from build123d import *

# Parameters (mm, degrees)
EXTRUDE_1_DEPTH     = 500
CUT_EXTRUDE_1_REACH = 4
SKETCH_2_R          = 3


with BuildPart() as part:
    # 草图1 → 凸台-拉伸1 (new body)
    with BuildSketch(Plane.XY):
        with BuildLine():
            Line((0, 0), (19.917157288, 0))
            ThreePointArc((19.917157288, 0), (19.993693974, 0.015224093), (20.058578644, 0.058578644))
            Line((20.058578644, 0.058578644), (43.444365081, 23.444365081))
            ThreePointArc((43.444365081, 23.444365081), (45, 24.088730163), (46.555634919, 23.444365081))
            Line((46.555634919, 23.444365081), (69.941421356, 0.058578644))
            ThreePointArc((69.941421356, 0.058578644), (70.006306026, 0.015224093), (70.082842712, 0))
            Line((70.082842712, 0), (90, 0))
            Line((90, 0), (90, -2))
            Line((90, -2), (70.082842712, -2))
            ThreePointArc((70.082842712, -2), (69.240939161, -1.832534972), (68.527207794, -1.355634919))
            Line((68.527207794, -1.355634919), (45.141421356, 22.030151519))
            ThreePointArc((45.141421356, 22.030151519), (45, 22.088730163), (44.858578644, 22.030151519))
            Line((44.858578644, 22.030151519), (21.472792206, -1.355634919))
            ThreePointArc((21.472792206, -1.355634919), (20.759060839, -1.832534972), (19.917157288, -2))
            Line((19.917157288, -2), (0, -2))
            Line((0, -2), (0, 0))
        make_face()
    extrude(amount=EXTRUDE_1_DEPTH)

    # 草图2 → 切除-拉伸1 (cut, up to next)
    with BuildSketch(Plane(origin=(0, 0, 0), x_dir=(1, 0, 0), z_dir=(0, 1, 0)), mode=Mode.PRIVATE) as cut_extrude_1_sk1:
        with Locations((9.958578644, -20)):
            Circle(SKETCH_2_R)
    cut_extrude_1_tool1 = extrude(cut_extrude_1_sk1.sketch, amount=-CUT_EXTRUDE_1_REACH, mode=Mode.PRIVATE) & part.part
    add(cut_extrude_1_tool1.solids().sort_by_distance((9.958579, 0, 20))[0], mode=Mode.SUBTRACT)
    # 草图2 → 切除-拉伸1 (cut, up to next)
    with BuildSketch(Plane(origin=(0, 0, 0), x_dir=(1, 0, 0), z_dir=(0, 1, 0)), mode=Mode.PRIVATE) as cut_extrude_1_sk2:
        with Locations((80.041421356, -20)):
            Circle(SKETCH_2_R)
    cut_extrude_1_tool2 = extrude(cut_extrude_1_sk2.sketch, amount=-CUT_EXTRUDE_1_REACH, mode=Mode.PRIVATE) & part.part
    add(cut_extrude_1_tool2.solids().sort_by_distance((80.041421, 0, 20))[0], mode=Mode.SUBTRACT)
    # 草图2 → 切除-拉伸1 (cut, up to next)
    with BuildSketch(Plane(origin=(0, 0, 0), x_dir=(1, 0, 0), z_dir=(0, 1, 0)), mode=Mode.PRIVATE) as cut_extrude_1_sk3:
        with Locations((9.958578644, -250)):
            Circle(SKETCH_2_R)
    cut_extrude_1_tool3 = extrude(cut_extrude_1_sk3.sketch, amount=-CUT_EXTRUDE_1_REACH, mode=Mode.PRIVATE) & part.part
    add(cut_extrude_1_tool3.solids().sort_by_distance((9.958579, 0, 250))[0], mode=Mode.SUBTRACT)
    # 草图2 → 切除-拉伸1 (cut, up to next)
    with BuildSketch(Plane(origin=(0, 0, 0), x_dir=(1, 0, 0), z_dir=(0, 1, 0)), mode=Mode.PRIVATE) as cut_extrude_1_sk4:
        with Locations((80.041421356, -250)):
            Circle(SKETCH_2_R)
    cut_extrude_1_tool4 = extrude(cut_extrude_1_sk4.sketch, amount=-CUT_EXTRUDE_1_REACH, mode=Mode.PRIVATE) & part.part
    add(cut_extrude_1_tool4.solids().sort_by_distance((80.041421, 0, 250))[0], mode=Mode.SUBTRACT)
    # 草图2 → 切除-拉伸1 (cut, up to next)
    with BuildSketch(Plane(origin=(0, 0, 0), x_dir=(1, 0, 0), z_dir=(0, 1, 0)), mode=Mode.PRIVATE) as cut_extrude_1_sk5:
        with Locations((9.958578644, -480)):
            Circle(SKETCH_2_R)
    cut_extrude_1_tool5 = extrude(cut_extrude_1_sk5.sketch, amount=-CUT_EXTRUDE_1_REACH, mode=Mode.PRIVATE) & part.part
    add(cut_extrude_1_tool5.solids().sort_by_distance((9.958579, 0, 480))[0], mode=Mode.SUBTRACT)
    # 草图2 → 切除-拉伸1 (cut, up to next)
    with BuildSketch(Plane(origin=(0, 0, 0), x_dir=(1, 0, 0), z_dir=(0, 1, 0)), mode=Mode.PRIVATE) as cut_extrude_1_sk6:
        with Locations((80.041421356, -480)):
            Circle(SKETCH_2_R)
    cut_extrude_1_tool6 = extrude(cut_extrude_1_sk6.sketch, amount=-CUT_EXTRUDE_1_REACH, mode=Mode.PRIVATE) & part.part
    add(cut_extrude_1_tool6.solids().sort_by_distance((80.041421, 0, 480))[0], mode=Mode.SUBTRACT)


solid = part.part
Input: part model. Units: mm. Frame: model coordinates. A direction names the side the tool comes from. Coordinates: 2 decimals unless noted, no trailing zeros. Write each loop counter-clockwise with the first axis right and the second up, starting at its lowest first coordinate (ties: lowest second). Pieces come first, ordered by that corner, then holes. Notation, with made-up numbers: M -21,37 L 33,37 A33 ccw 33,70 Z; hole C -4,76 d8. An arc over 180 degrees is marked long. Answer as a JSON object with one key per item and string values. Group by question number.
(1) Contact query for flat-ended pins moving along their axis: P1, Ø4, axis at x = 38, z = 338, coming from the +Y side; P2, Ø22, axis at x = 6.5, z = 287, coming from the +Y side; P3, Ø4, axis at y = 15.5, z = 81.5, coming from the -X side. Output: stop coordinate, or through.
(2) Ray query, line 1 along X through (y, z) = (-1.3, 250); line 2 along X through (y, z) = (-1.25, 20); line 3 along Y through (x, z) = (6, 291.5). Return the intervals inside material, ascending. Write a range as [from, to].
(3) Set-up query: faces 4 (the face through (10, 0, 246)), 5 (the face through (57, 10.17, 246.5)), 6 (the face through (80, 0, 246)). Return all of +Z, -Z, +X, -X, +Y, -Y with unobstructed straight access to the full face (end or side cutting, diameter ignored); none if empty.
(4) Section A-A on y = 13.5. Output: boundary loops of the cut face in (x, z).
(5) Mould query, pull axis X, two halves, no side actions, for faces 1 (the face through (58, 12, 246)), 2 (the face through (33.33, 10.5, 246.5)), 3 (the face through (80, -2, 246)). Classes: pulls with the +X half, pulls with the -X half, needs draft (parallel to the pull), parting line crosses it, or undercut.
(6) Section B-B on z = 205.5. Output: boundary loops of the cut face in (x, y).
Result set:
{
 "1": {"P1": "stops at y = 20", "P2": "stops at y = 0", "P3": "stops at x = 33.5"},
 "2": {"line 1": "x = [0, 6.96], [12.96, 21.53], [68.47, 77.04], [83.04, 90]", "line 2": "x = [0, 6.96], [12.96, 21.58], [68.42, 77.04], [83.04, 90]", "line 3": "y = [-2, 0]"},
 "3": {"face 4": "+Z, -Z, -X, +Y", "face 5": "+Z, -Z, -Y", "face 6": "+Z, -Z, +X, +Y"},
 "4": {"outline": "M 33.5,0 L 36.33,0 L 36.33,500 L 33.5,500 Z; M 53.67,0 L 56.5,0 L 56.5,500 L 53.67,500 Z"},
 "5": {"face 1": "pulls with the +X half", "face 2": "undercut", "face 3": "needs draft"},
 "6": {"outline": "M 0,-2 L 19.92,-2 A2.2 ccw 21.47,-1.36 L 44.86,22.03 A0.2 cw 45.14,22.03 L 68.53,-1.36 A2.2 ccw 70.08,-2 L 90,-2 L 90,0 L 70.08,0 A0.2 cw 69.94,0.06 L 46.56,23.44 A2.2 ccw 43.44,23.44 L 20.06,0.06 A0.2 cw 19.92,0 L 0,0 Z"}
}
